```python
from build123d import *

# Parameters (mm, degrees)
SKETCH1_W           = 20
SKETCH1_H           = 86
BOSS_EXTRUDE1_DEPTH = 4.9
BOSS_EXTRUDE4_DEPTH = 40
SKETCH2_R           = 1.95
CUT_EXTRUDE1_DEPTH  = 6


with BuildPart() as part:
    # Sketch1 → Boss-Extrude1 (new body)
    with BuildSketch(Plane(origin=(0, 0, 0), x_dir=(1, 0, 0), z_dir=(0, 1, 0))):
        Rectangle(SKETCH1_W, SKETCH1_H)
    extrude(amount=BOSS_EXTRUDE1_DEPTH)

    # Sketch4 → Boss-Extrude4 (add)
    with BuildSketch(Plane.XY.offset(43)):
        Polygon((-3.9, 0), (-3.9, -4.2), (-6.8, -4.2), (-3.9, -8), (3.9, -8), (6.8, -4.2), (3.9, -4.2), (3.9, 0), align=None)
    extrude(amount=-BOSS_EXTRUDE4_DEPTH)

    # Sketch2 → Cut-Extrude1 (cut)
    with BuildSketch(Plane(origin=(0, 4.9, 0), x_dir=(1, 0, 0), z_dir=(0, 1, 0))):
        with Locations((1.5, -39.5)):
            Circle(SKETCH2_R)
        with Locations((1.5, 39.5)):
            Circle(SKETCH2_R)
    extrude(amount=-CUT_EXTRUDE1_DEPTH, mode=Mode.SUBTRACT)


solid = part.part
```
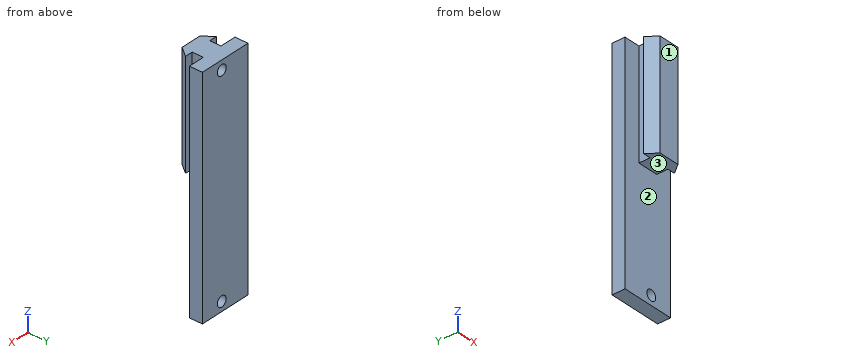
Check sheet for the modelled part. Datum: model origin and axes. Units: mm. Face numbers are marked on the shaded views. Coordinates: 2 decimals unless noted, no trailing zeros. Write each loop counter-clockwise with the first axis right and the second up, starting at its lowest first coordinate (ties: lowest second). Pieces come first, ordered by that corner, then holes. Notation, with made-up numbers: (-12, -33.75) - (10, -33.75) arc R26 ccw to (10, -14.75) - close; hole circle Ø3 at (44.5, -1.75). An arc over 180 degrees is marked (long way). One line per question, with ' | ' between items.
Item 1: Thickness scan on line 1 (Z direction, x = 1.5, y = 2.55); line 2 (X direction, y = 2.8, z = -39.5); line 3 (Y direction, x = 7, z = 25). Record the ranges inside material, lowest first. Write a range as [from, to].
Determined:
line 1: z = [-43, -41.45], [-37.55, 37.55], [41.45, 43] | line 2: x = [-10, -0.45], [3.45, 10] | line 3: y = [0, 4.9]
Item 2: Sectioned sample at C-C on z = 39.5. Record the boundary of the cut face in (x, y).
Determined:
outline: (-10, 0) - (-3.9, 0) - (-3.9, -4.2) - (-6.8, -4.2) - (-3.9, -8) - (3.9, -8) - (6.8, -4.2) - (3.9, -4.2) - (3.9, 0) - (10, 0) - (10, 4.9) - (3.45, 4.9) - (3.45, -1.1) - (-0.45, -1.1) - (-0.45, 4.9) - (-10, 4.9) - close
Item 3: Gauge pin test, flat ends, axial feed: P1, Ø3.5, axis at x = 1.5, z = 39.5, coming from the +Y side; P2, Ø6, axis at x = 1.5, z = -39.5, coming from the -Y side; P3, Ø3.5, axis at y = -3, z = 21, coming from the +X side. Record the tip position at first contact, or that the pin passes through.
Determined:
P1: stops at y = -1.1 | P2: stops at y = 0 | P3: stops at x = 6.8
Item 4: Mould release check, pull along Y, two halves, no side actions. Record for the marked faces 1, 2 and 3: pulls with the +Y half, pulls with the -Y half, needs draft (parallel to the pull), parting line crosses it, or undercut.
Determined:
face 1: pulls with the -Y half | face 2: undercut | face 3: needs draft
Item 5: Sectioned sample at D-D on x = 8.5. Record the boundary of the cut face in (y, z).
Determined:
outline: (0, -43) - (4.9, -43) - (4.9, 43) - (0, 43) - close
Item 6: Sectioned sample at B-B on x = 1.5. Record the boundary of the cut face in (y, z).
Determined:
outline: (-8, 3) - (0, 3) - (0, -37.55) - (4.9, -37.55) - (4.9, 37.55) - (-1.1, 37.55) - (-1.1, 41.45) - (4.9, 41.45) - (4.9, 43) - (-8, 43) - close; (0, -43) - (4.9, -43) - (4.9, -41.45) - (0, -41.45) - close
Item 7: Sectioned sample at A-A on z = -39.5. Record the boundary of the cut face in (x, y), plus the area to 3 significant figures.
Determined:
outline: (-10, 0) - (-0.45, 0) - (-0.45, 4.9) - (-10, 4.9) - close; (3.45, 0) - (10, 0) - (10, 4.9) - (3.45, 4.9) - close | area: 78.9 mm2
